Check sheet for the modelled part. Datum: model origin and axes. Units: mm. A direction names the side the tool comes from. Give positions to 0.01 mm unless a question says otherwise; leave off trailing zeros. Order: outer loops, then holes, each group sorted by start corner. A loop starts at its lowest first (then second) coordinate and runs counter-clockwise, first axis right, second up.
from build123d import *

# Parameters (mm, degrees)
SKETCH1_R           = 3
BOSS_EXTRUDE1_DEPTH = 30
SKETCH2_R           = 5
BOSS_EXTRUDE2_DEPTH = 0.5
BOSS_EXTRUDE3_DEPTH = 3
CHAMFER1_SIZE       = 0.5
CHAMFER2_SIZE       = 0.25


with BuildPart() as part:
    # Sketch1 → Boss-Extrude1 (new body)
    with BuildSketch(Plane.XY):
        Circle(SKETCH1_R)
    extrude(amount=BOSS_EXTRUDE1_DEPTH)

    # Sketch2 → Boss-Extrude2 (add)
    with BuildSketch(Plane.XY.offset(30)):
        Circle(SKETCH2_R)
    extrude(amount=BOSS_EXTRUDE2_DEPTH)

    # Sketch3 → Boss-Extrude3 (add)
    with BuildSketch(Plane.XY.offset(30.5)):
        Polygon((5.773502692, 0), (2.886751346, 5), (-2.886751346, 5), (-5.773502692, 0), (-2.886751346, -5), (2.886751346, -5), align=None)
    extrude(amount=BOSS_EXTRUDE3_DEPTH)

    # Chamfer1
    chamfer1_edges = [part.edges().sort_by_distance(p)[0] for p in [
        (-3, 0, 0),
    ]]
    chamfer(chamfer1_edges, length=CHAMFER1_SIZE)

    # Chamfer2
    chamfer2_edges = [part.edges().sort_by_distance(p)[0] for p in [
        (-3, 0, 30),
    ]]
    chamfer(chamfer2_edges, length=CHAMFER2_SIZE)


solid = part.part
1) Material ranges on L1, parallel to Z at x = -3.25, y = 3; L2, parallel to X at y = -0.5, z = 9.5; L3, parallel to X at y = -1.5, z = 15.5, recorded low to high.
Recorded:
L1: z = 30 to 33.5
L2: x = -2.96 to 2.96
L3: x = -2.6 to 2.6
2) Depth check by flat-ended pin: pin 1 Ø1.2 at (x, y) = (5, 0.5) entering from -Z; pin 2 Ø2 at (y, z) = (0, 19.5) entering from -X; pin 3 Ø3 at (x, z) = (-2, 14) entering from -Y. Enter the tip coordinate at first touch or a pass-through.
Recorded:
pin 1: stops at z = 30
pin 2: stops at x = -3
pin 3: stops at y = -2.96
3) Section check A-A, the plane z = 17.5. Record the cut outline in (x, y), then the cut area to 3 significant figures.
Recorded:
outline: circle Ø6 at (0, 0)
area: 28.3 mm2
4) Set-up check for faces 1 (the face through (-2.7, 4.5, 30.5)), 2 (the face through (2.6, -4.5, 30.5)), 3 (the face through (2.6, 4.5, 30.5)), 4 (the face through (-1.08, -4.88, 30.25)), 5 (the face through (-2.7, -4.5, 30.5)): record each of +Z, -Z, +X, -X, +Y, -Y from which the full face is reachable in a straight line by a thin tool's end or side.
Recorded:
face 1: -Z, -X, +Y
face 2: -Z, +X, -Y
face 3: -Z, +X, +Y
face 4: -Z
face 5: -Z, -X, -Y
